Input: part model. Units: mm. Frame: model coordinates. Give positions to 0.01 mm unless a question says otherwise; leave off trailing zeros. Loops run counter-clockwise (first coordinate to the right, second up) from the corner with the lowest first, then second, coordinate; pieces in that order, holes last. Notation, with made-up numbers: (64, -37) -> (83, -37) arc R33 cw to (83, 1) -> close; hole circle Ø1 at (-12, -27). An arc over 180 degrees is marked (long way). One line per question, with ' | ' between items.
from build123d import *

# Parameters (mm, degrees)
SKETCH018_R  = 200
PAD011_DEPTH = 395
SKETCH016_R  = 59
PAD010_DEPTH = 11
SKETCH015_R  = 60
PAD009_DEPTH = 11


with BuildPart() as pad011:
    # Sketch018 → Pad011 (new body)
    with BuildSketch(Plane.XY.offset(-11)):
        Circle(SKETCH018_R)
    extrude(amount=PAD011_DEPTH)


with BuildPart() as cut010:
    # Sphere → Sphere (revolve)
    with BuildSketch(Plane(origin=(0, 0, 116), x_dir=(1, 0, 0), z_dir=(0, -1, 0))):
        with BuildLine():
            ThreePointArc((0, -140.5), (140.5, 0), (0, 140.5))
            Line((0, 140.5), (0, -140.5))
        make_face()
    revolve(axis=Axis((0, 0, 116), (0, 0, 1)))

    # Cut010: cut Pad011
    add(pad011.part, mode=Mode.SUBTRACT)


with BuildPart() as pad010:
    # Sketch016 → Pad010 (new body)
    with BuildSketch(Plane.XY):
        Circle(SKETCH016_R)
    extrude(amount=-PAD010_DEPTH)


with BuildPart() as fusion:
    # Sketch015 → Pad009 (new body)
    with BuildSketch(Plane.XY):
        Circle(SKETCH015_R)
    extrude(amount=-PAD009_DEPTH)

    # Cut006: cut Pad010
    add(pad010.part, mode=Mode.SUBTRACT)

    # Fusion: union Cut010
    add(cut010.part)


solid = fusion.part
1. Section query A-A (y = 0). Output: boundary loops of the cut face in (x, z).
Determined:
outline: (-60.09, -11) arc R140.5 ccw to (60.09, -11) -> (60, -11) -> (60, 0) -> (59, 0) -> (59, -11) -> (-59, -11) -> (-59, 0) -> (-60, 0) -> (-60, -11) -> close
2. Ray query, line 1 along Y through (x, z) = (0, -8); line 2 along Y through (x, z) = (36.5, -7.75); line 3 along X through (y, z) = (45, -10.25). Return the intervals inside material, ascending. Write a range as from..to.
Determined:
line 1: y = -60..-59, 59..60 | line 2: y = -47.62..-46.35, 46.35..47.62 | line 3: x = -39.69..-38.16, 38.16..39.69
3. Section query D-D (z = -20.25). Output: boundary loops of the cut face in (x, y).
Determined:
outline: circle Ø68.59 at (0, 0)
4. Pull-direction query (Y, two-part tool) for faces 1 (the flat face through (44, -40, 0)), 2 (the cylindrical face through (56.275, 17.722, -5.423)), 3 (the cylindrical face through (-59.94, 2.64, -5.42)); classes: pulls with the +Y half, pulls with the -Y half, needs draft (parallel to the pull), parting line crosses it, or undercut.
Determined:
face 1: needs draft | face 2: undercut | face 3: parting line crosses it
5. Pin query (flat end, axial travel): P1, Ø2, axis at x = -47.5, z = -11.5, coming from the +Y side; P2, Ø4, axis at y = 37.5, z = -5, coming from the -X side; P3, Ø3, axis at y = -0.5, z = -4, coming from the -X side. Return the tip coordinate at first contact, or that it passes through.
Determined:
P1: stops at y = 37.9 | P2: stops at x = -48.37 | P3: stops at x = -60
6. Section query C-C (z = -9). Output: boundary loops of the cut face in (x, y).
Determined:
outline: circle Ø120 at (0, 0); hole circle Ø118 at (0, 0)
